Autodesk Inventor part; units mm, degrees
ref_plane "YZ Plane" through (0, 0, 0) normal (1, 0, 0) x (0, 1, 0)
ref_plane "XZ Plane" through (0, 0, 0) normal (0, 1, 0) x (-1, 0, 0)
ref_plane "XY Plane" through (0, 0, 0) normal (0, 0, 1) x (1, 0, 0)
sketch "Skizze1" plane through (0, 0, 0) normal (0, 0, 1) x (1, 0, 0)
  line L0 (0, 0) -> (85, 0)
  line L1 (85, 0) -> (85, 80)
  line L2 (85, 80) -> (0, 80)
  line L3 (0, 80) -> (0, 0)
  dimension "d0" = 85
  dimension "d1" = 80
extrude "Extrusion1" add sketch "Skizze1" along normal blind 5
sketch "Skizze3" plane through (0, 0, 5) normal (0, 0, 1) x (1, 0, 0)
  line L0 (7.5, 71) -> (77.5, 71)
  line L1 (77.5, 71) -> (77.5, 9)
  line L2 (77.5, 9) -> (7.5, 9)
  line L3 (7.5, 9) -> (7.5, 71)
  line L4 (85, 80) -> (0, 80)
  line L5 (85, 0) -> (85, 80)
  line L6 (16.85, 66.85) -> (68.15, 66.85)
  line L7 (68.15, 66.85) -> (68.15, 42.15)
  line L8 (68.15, 42.15) -> (16.85, 42.15)
  line L9 (16.85, 42.15) -> (16.85, 66.85)
  line L10 (10.5, 37.5) -> (20.5, 37.5)
  line L11 (20.5, 37.5) -> (20.5, 27.5)
  line L12 (20.5, 27.5) -> (10.5, 27.5)
  line L13 (10.5, 27.5) -> (10.5, 37.5)
  line L14 (15.5, 37.5) -> (15.5, 27.5)
  line L15 (10.5, 32.5) -> (20.5, 32.5)
  line L16 (24.5, 37.5) -> (34.5, 37.5)
  line L17 (34.5, 37.5) -> (34.5, 27.5)
  line L18 (34.5, 27.5) -> (24.5, 27.5)
  line L19 (24.5, 27.5) -> (24.5, 37.5)
  line L20 (38.5, 37.5) -> (48.5, 37.5)
  line L21 (48.5, 37.5) -> (48.5, 27.5)
  line L22 (48.5, 27.5) -> (38.5, 27.5)
  line L23 (38.5, 27.5) -> (38.5, 37.5)
  line L24 (52.5, 37.5) -> (62.5, 37.5)
  line L25 (62.5, 37.5) -> (62.5, 27.5)
  line L26 (62.5, 27.5) -> (52.5, 27.5)
  line L27 (52.5, 27.5) -> (52.5, 37.5)
  line L28 (66.5, 37.5) -> (76.5, 37.5)
  line L29 (76.5, 37.5) -> (76.5, 27.5)
  line L30 (76.5, 27.5) -> (66.5, 27.5)
  line L31 (66.5, 27.5) -> (66.5, 37.5)
  point P0 (0, 0)
  point P1 (77.5, 40)
  point P2 (85, 40)
  point P3 (42.5, 71)
  point P4 (42.5, 80)
  point P5 (42.5, 66.85)
  dimension "d9" = 70
  dimension "d10" = 62
  dimension "d12" = 51.3
  dimension "d13" = 24.7
  dimension "d14" = 4.15
  dimension "d15" = 10
  dimension "d16" = 10
  dimension "d21" = 8
  dimension "d22" = 23.5
  dimension "d23" = 14
  dimension "d24" = 14
  dimension "d25" = 14
  dimension "d26" = 14
extrude "Extrusion3" cut sketch "Skizze3" against normal through all contours L6 L7 L8 L9 | L10 L14 L15 L13 | L10 L11 L15 L14 | L15 L14 L12 L13 | L15 L11 L12 L14 | L16 L17 L18 L19 | L20 L21 L22 L23 | L24 L25 L26 L27 | L28 L29 L30 L31
sketch "Skizze5" plane through (0, 0, 0) normal (0, 0, -1) x (-1, 0, 0)
  line L0 (-20.5, 27.5) -> (-20.5, 37.5)
  line L1 (-20.5, 37.5) -> (-10.5, 37.5)
  line L2 (-10.5, 37.5) -> (-10.5, 27.5)
  line L3 (-10.5, 27.5) -> (-20.5, 27.5)
  line L4 (-66.5, 37.5) -> (-66.5, 27.5)
  line L5 (-66.5, 27.5) -> (-76.5, 27.5)
  line L6 (-76.5, 27.5) -> (-76.5, 37.5)
  line L7 (-76.5, 37.5) -> (-66.5, 37.5)
  line L8 (-38.5, 37.5) -> (-38.5, 27.5)
  line L9 (-38.5, 27.5) -> (-48.5, 27.5)
  line L10 (-48.5, 27.5) -> (-48.5, 37.5)
  line L11 (-48.5, 37.5) -> (-38.5, 37.5)
  line L12 (-24.5, 37.5) -> (-24.5, 27.5)
  line L13 (-24.5, 27.5) -> (-34.5, 27.5)
  line L14 (-34.5, 27.5) -> (-34.5, 37.5)
  line L15 (-34.5, 37.5) -> (-24.5, 37.5)
  line L16 (-52.5, 37.5) -> (-52.5, 27.5)
  line L17 (-52.5, 27.5) -> (-62.5, 27.5)
  line L18 (-62.5, 27.5) -> (-62.5, 37.5)
  line L19 (-62.5, 37.5) -> (-52.5, 37.5)
  line L20 (-16.85, 66.85) -> (-16.85, 42.15)
  line L21 (-16.85, 42.15) -> (-68.15, 42.15)
  line L22 (-68.15, 42.15) -> (-68.15, 66.85)
  line L23 (-68.15, 66.85) -> (-16.85, 66.85)
  line L24 (0, 0) -> (-85, 0)
  line L25 (0, 80) -> (0, 0)
  line L26 (-85, 80) -> (0, 80)
  line L27 (-85, 0) -> (-85, 80)
  line L28 (-4, 76) -> (-4, 4)
  line L29 (-4, 4) -> (-81, 4)
  line L30 (-81, 4) -> (-81, 76)
  line L31 (-81, 76) -> (-4, 76)
  line L32 (-85, 80) -> (0, 80)
  dimension "d39" = 4
hole "Bohrung2" at (4, 76, 0) at (4, 4, 0) at (81, 4, 0) at (81, 76, 0) direction (0, 0, 1) diameter 4.5 end through all
sketch "Skizze6" plane through (0, 0, 0) normal (0, 0, -1) x (-1, 0, 0)
  circle A0 centre (-15.65, 22.5) radius 2.45
  circle A1 centre (-29.65, 22.5) radius 2.45
  circle A2 centre (-43.65, 22.5) radius 2.45
  point P0 (0, 0)
hole "Bohrung3" at (43.65, 22.5, 0) at (29.65, 22.5, 0) at (15.65, 22.5, 0) direction (0, 0, 1) diameter 5 end through all
fillet "Rundung2" radius 2 4 edges at (85, 0, 2.5) (0, 0, 2.5) (0, 80, 2.5) (85, 80, 2.5)
fillet "Rundung1" radius 2.1 24 edges at (10.5, 37.5, 2.5) (10.5, 27.5, 2.5) (20.5, 27.5, 2.5) (20.5, 37.5, 2.5) (24.5, 37.5, 2.5) (24.5, 27.5, 2.5) (34.5, 27.5, 2.5) (34.5, 37.5, 2.5) (38.5, 37.5, 2.5) (48.5, 37.5, 2.5) (52.5, 37.5, 2.5) (62.5, 37.5, 2.5) (66.5, 37.5, 2.5) (76.5, 37.5, 2.5) (76.5, 27.5, 2.5) (66.5, 27.5, 2.5) (62.5, 27.5, 2.5) (52.5, 27.5, 2.5) (48.5, 27.5, 2.5) (38.5, 27.5, 2.5) (16.85, 42.15, 2.5) (16.85, 66.85, 2.5) (68.15, 66.85, 2.5) (68.15, 42.15, 2.5)
properties part number "Schiled"
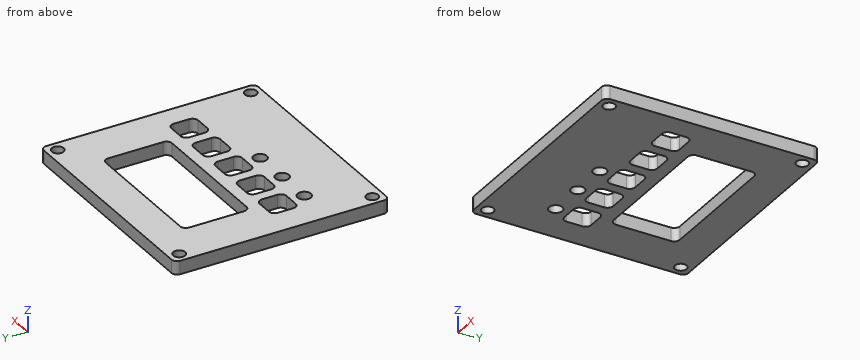
CAD build for the part. Positions are in the model's coordinates, mm. Round coordinates to 2 decimals unless told otherwise and drop trailing zeros. Write each loop counter-clockwise with the first axis right and the second up, starting at its lowest first coordinate (ties: lowest second). Pieces come first, ordered by that corner, then holes.
Item 1: Band-saw the part on A-A on x = 65. Write the cut outline in (y, z).
Filled in:
outline: (0, 0) - (42.15, 0) - (42.15, 5) - (0, 5) - close; (66.85, 0) - (80, 0) - (80, 5) - (66.85, 5) - close
Item 2: Band-saw the part on D-D on x = 29.65. Write the cut outline in (y, z).
Filled in:
outline: (0, 0) - (20, 0) - (20, 5) - (0, 5) - close; (25, 0) - (27.5, 0) - (27.5, 5) - (25, 5) - close; (37.5, 0) - (42.15, 0) - (42.15, 5) - (37.5, 5) - close; (66.85, 0) - (80, 0) - (80, 5) - (66.85, 5) - close
Item 3: Band-saw the part on C-C on x = 15.65. Write the cut outline in (y, z), then the cut area to 3 significant figures.
Filled in:
outline: (0, 0) - (20, 0) - (20, 5) - (0, 5) - close; (25, 0) - (27.5, 0) - (27.5, 5) - (25, 5) - close; (37.5, 0) - (80, 0) - (80, 5) - (37.5, 5) - close
area: 325 mm2
Item 4: Band-saw the part on B-B on y = 76. Write the cut outline in (x, z).
Filled in:
outline: (0, 0) - (1.75, 0) - (1.75, 5) - (0, 5) - close; (6.25, 0) - (78.75, 0) - (78.75, 5) - (6.25, 5) - close; (83.25, 0) - (85, 0) - (85, 5) - (83.25, 5) - close
Item 5: Drill centre lines: L1, parallel to Y at x = 81, z = 2.7; L2, parallel to Y at x = 41, z = 0.45; L3, parallel to X at y = 22.5, z = 2.8. Where is each one in solid material? Low to high.
Filled in:
L1: y = 0 to 1.75, 6.25 to 73.75, 78.25 to 80
L2: y = 0 to 27.5, 37.5 to 42.15, 66.85 to 80
L3: x = 0 to 13.15, 18.15 to 27.15, 32.15 to 41.15, 46.15 to 85
